Job drawing, mm, ordinate dimensions from the low corner. One solid piece. A direction names the side the tool comes from. Give positions to 0.01 mm unless a question says otherwise; leave off trailing zeros. Loops run counter-clockwise (first coordinate to the right, second up) from the corner with the lowest first, then second, coordinate; pieces in that order, holes last. Notation, with made-up numbers: M -38.75,4.25 L 12.25,4.25 A9 cw 12.25,19.25 Z; hole C 69.5,-34 d4. An arc over 180 degrees is marked long. Answer in a Markdown table with one row per item.
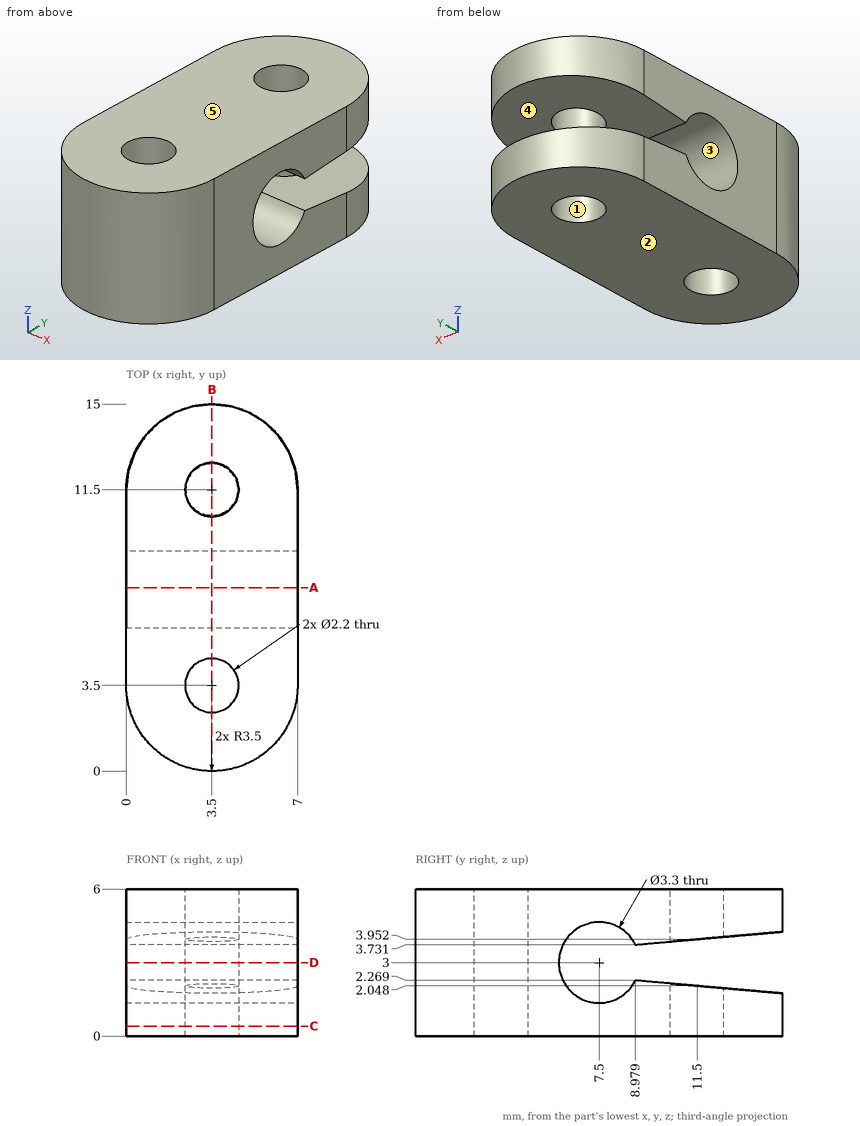
(1) Saw through at C-C (z = 0.4). Write the cut outline in (x, y).
Recorded:
| item | result |
|---|---|
| outline | M 0,3.5 A3.5 ccw 7,3.5 L 7,11.5 A3.5 ccw 0,11.5 Z; hole C 3.5,3.5 d2.2; hole C 3.5,11.5 d2.2 |
(2) Which spindle directions (+Z, -Z, +X, -X, +Y, -Y) get a long thin tool onto all of the face, cutting with end or side? Do the marked faces 4 and 5. Say none if no direction does.
Recorded:
| item | result |
|---|---|
| face 4 | +X, -X, +Y |
| face 5 | +Z, +X, -X, +Y, -Y |
(3) Saw through at B-B (x = 3.5). Give the number of separate pieces and of enclosed holes in the cut face.
Recorded:
| item | result |
|---|---|
| separate pieces | 4 |
| enclosed holes | 0 |
(4) Pull direction Z, two halves, no side cores. Call the marked faces 1, 2 and 3: +Z half, -Z half, draft (parallel to the pull), parting line (faces both ways), or undercut.
Recorded:
| item | result |
|---|---|
| face 1 | draft |
| face 2 | -Z half |
| face 3 | undercut |
(5) Saw through at D-D (z = 3). Write the cut outline in (x, y).
Recorded:
| item | result |
|---|---|
| outline | M 0,3.5 A3.5 ccw 7,3.5 L 7,5.85 L 0,5.85 Z; hole C 3.5,3.5 d2.2 |
(6) Saw through at A-A (y = 7.5). Write the cut outline in (x, z), plus the area to 3 significant figures.
Recorded:
| item | result |
|---|---|
| outline | M 0,0 L 7,0 L 7,1.35 L 0,1.35 Z; M 0,4.65 L 7,4.65 L 7,6 L 0,6 Z |
| area | 18.9 mm^2 |
(7) Drill centre lines: line 1 along Y through (x, z) = (3.5, 1.25); line 2 along Y through (x, z) = (2.75, 0.6) (1 decimal); line 3 along Z through (x, y) = (4, 7.5). Where is each one in solid material? Low to high.
Recorded:
| item | result |
|---|---|
| line 1 | y = 0 to 2.4, 4.6 to 10.4, 12.6 to 15 |
| line 2 | y = 0.1 to 2.7, 4.3 to 10.7, 12.3 to 14.9 |
| line 3 | z = 0 to 1.35, 4.65 to 6 |
